Design review of the part built by this model. Coordinates are the model's own, in mm. A direction names the side the tool comes from. Give positions to 0.01 mm unless a question says otherwise; leave off trailing zeros. Write each loop counter-clockwise with the first axis right and the second up, starting at its lowest first coordinate (ties: lowest second). Pieces come first, ordered by that corner, then holes.
```python
from build123d import *

# Parameters (mm, degrees)
SKETCH_1_W          = 10
SKETCH_1_H          = 10
EXTRUDE_1_DEPTH     = 1
SKETCH_2_W          = 25
SKETCH_2_H          = 2
EXTRUDE_2_DEPTH     = 1
SKETCH_3_W          = 25
SKETCH_3_H          = 2
EXTRUDE_3_DEPTH     = 1
SKETCH_4_R          = 2.5
EXTRUDE_4_DEPTH     = 8
SKETCH_5_R          = 2.5
SKETCH_5_R_2        = 0.5
CUT_EXTRUDE_3_DEPTH = 1
CUT_EXTRUDE_START   = -1
SKETCH_6_R          = 2.5
SKETCH_6_R_2        = 0.5
CUT_EXTRUDE_4_DEPTH = 1


with BuildPart() as part:
    # 草图1 → 凸台-拉伸1 (new body)
    with BuildSketch(Plane(origin=(0, 0, 0), x_dir=(0, 0, -1), z_dir=(1, 0, 0))):
        with Locations((5, 5)):
            Rectangle(SKETCH_1_W, SKETCH_1_H)
    extrude(amount=EXTRUDE_1_DEPTH)

    # 草图2 → 凸台-拉伸2 (add)
    with BuildSketch(Plane.XY):
        with Locations((13.5, 5)):
            Rectangle(SKETCH_2_W, SKETCH_2_H)
    extrude(amount=-EXTRUDE_2_DEPTH)

    # 草图3 → 凸台-拉伸3 (add)
    with BuildSketch(Plane(origin=(0, 0, -10), x_dir=(-1, 0, 0), z_dir=(0, 0, -1))):
        with Locations((-13.5, 5)):
            Rectangle(SKETCH_3_W, SKETCH_3_H)
    extrude(amount=-EXTRUDE_3_DEPTH)

    # 草图4 → 凸台-拉伸4 (add)
    with BuildSketch(Plane(origin=(0, 0, -1), x_dir=(-1, 0, 0), z_dir=(0, 0, -1))):
        with Locations(Location((-23, 5, 0), (0, 0, 203.578178478))):
            Circle(SKETCH_4_R)
    extrude(amount=EXTRUDE_4_DEPTH)

    # 草图5 → 切除-拉伸3 (cut)
    with BuildSketch(Plane.XY.offset(-1)):
        with Locations((23, 5)):
            Circle(SKETCH_5_R)
        with Locations((23, 5)):
            Circle(SKETCH_5_R_2, mode=Mode.SUBTRACT)
    extrude(amount=-CUT_EXTRUDE_3_DEPTH, mode=Mode.SUBTRACT)

    # 草图6 → 切除-拉伸4 (cut)
    with BuildSketch(Plane(origin=(0, 0, -9), x_dir=(-1, 0, 0), z_dir=(0, 0, -1)).offset(CUT_EXTRUDE_START)):
        with Locations(Location((-23, 5, 0), (0, 0, 180))):
            Circle(SKETCH_6_R)
        with Locations(Location((-23, 5, 0), (0, 0, 180))):
            Circle(SKETCH_6_R_2, mode=Mode.SUBTRACT)
    extrude(amount=CUT_EXTRUDE_4_DEPTH, mode=Mode.SUBTRACT)


solid = part.part
```
(1) Consider section C-C, the plane z = -6.5. Give the boundary of the cut face in (x, y), then the cut area to 3 significant figures.
Resolved:
outline: (0, 0) - (1, 0) - (1, 10) - (0, 10) - close; circle Ø5 at (23, 5)
area: 29.6 mm2
(2) Consider section D-D, the plane x = 23. Give the boundary of the cut face in (y, z), then the cut area to 3 significant figures.
Resolved:
outline: (2.5, -8) - (4.5, -8) - (4.5, -9) - (4, -9) - (4, -10) - (6, -10) - (6, -9) - (5.5, -9) - (5.5, -8) - (7.5, -8) - (7.5, -2) - (5.5, -2) - (5.5, -1) - (6, -1) - (6, 0) - (4, 0) - (4, -1) - (4.5, -1) - (4.5, -2) - (2.5, -2) - close
area: 36.0 mm2
(3) Consider section A-A, the plane x = 8. Give the boundary of the cut face in (y, z), then the cut area to 3 significant figures.
Resolved:
outline: (4, -10) - (6, -10) - (6, -9) - (4, -9) - close; (4, -1) - (6, -1) - (6, 0) - (4, 0) - close
area: 4.00 mm2
(4) Tool access review of faces 1 (the face through (13.3, 6, -0.5)), 2 (the face through (13.3, 4, -0.5)), 3 (the face through (13.7, 4, -9.5)), 4 (the face through (23.477, 4.85, -8.493)), 5 (the face through (0.5, 0, -4.9)): name each direction out of +Z, -Z, +X, -X, +Y, -Y from which nothing blocks a thin tool from reaching the whole face with its end or side.
Resolved:
face 1: +Z, +X, +Y
face 2: +Z, +X, -Y
face 3: -Z, +X, -Y
face 4: none
face 5: +Z, -Z, +X, -X, -Y
(5) Clearance check with flat-ended pins moving along their axes: P1, Ø5, axis at x = 21.5, z = -5, coming from the +Y side; P2, Ø0.5, axis at x = 18.5, z = -0.5, coming from the +Y side; P3, Ø3, axis at y = 3.5, z = -5.5, coming from the +X side; P4, Ø1.5, axis at x = 10, y = 8.5, coming from the +Z side. State where each tip first meets the part, or that it passes through.
Resolved:
P1: stops at y = 7.5
P2: stops at y = 6
P3: stops at x = 25.5
P4: passes through
(6) To check wall thickness, follow L1, parallel to Z at x = 24.75, y = 4.75; L2, parallel to X at y = 8.5, z = -5.75; L3, parallel to Y at x = 24.25, z = -9.25. State the ranges of each line that lie inside material, in increasing order.
Resolved:
L1: z = -10 to -9, -8 to -2, -1 to 0
L2: x = 0 to 1
L3: y = 4 to 6
(7) Consider section B-B, the plane y = 5. Give the boundary of the cut face in (x, z).
Resolved:
outline: (0, -10) - (26, -10) - (26, -9) - (23.5, -9) - (23.5, -8) - (25.5, -8) - (25.5, -2) - (23.5, -2) - (23.5, -1) - (26, -1) - (26, 0) - (0, 0) - close; hole (1, -9) - (22.5, -9) - (22.5, -8) - (20.5, -8) - (20.5, -2) - (22.5, -2) - (22.5, -1) - (1, -1) - close
(8) Mouldability with a two-part tool opening along Z and no side actions: class faces 6 (the face through (13.7, 6, -9.5)), 7 (the face through (11, 5, 0)), 8 (the face through (20.667, 5.898, -4.958)), 9 (the face through (11, 5, -10)) as pulls with the +Z half, pulls with the -Z half, needs draft (parallel to the pull), parting line crosses it, or undercut.
Resolved:
face 6: needs draft
face 7: pulls with the +Z half
face 8: undercut
face 9: pulls with the -Z half
